```python
from build123d import *

# Parameters (mm, degrees)
SKIZZE2_R                            = 0.75
SCHNITT_LINEAR_AUSTRAGEN1_DEPTH      = 60.476886267
SKIZZE3_R                            = 3.5
SCHNITT_LINEAR_AUSTRAGEN2_DEPTH      = 25
SCHNITT_LINEAR_AUSTRAGEN3_DEPTH      = 60.476886267
SCHNITT_LINEAR_AUSTRAGEN3_DEPTH_BACK = 5
SKIZZE4_R                            = 6
SKIZZE5_W                            = 10
SKIZZE5_H                            = 60
SCHNITT_LINEAR_AUSTRAGEN4_DEPTH      = 60.476886435


with BuildPart() as part:
    # Skizze1 → Rotation1 (revolve)
    with BuildSketch(Plane.XY, mode=Mode.PRIVATE) as rotation1_sk:
        Polygon((0, 0), (-22.5, 0), (-27.5, 45), (0, 45), align=None)
    revolve(rotation1_sk.sketch.rotate(Axis((0, 0, 0), (0, 1, 0)), 270), axis=Axis((0, 0, 0), (0, 1, 0)))

    # Skizze2 → Schnitt-Linear austragen1 (cut, through all)
    with BuildSketch(Plane(origin=(0, 45, 0), x_dir=(1, 0, 0), z_dir=(0, 1, 0))):
        with Locations(Location((0, 0, 0), (0, 0, 270))):
            Circle(SKIZZE2_R)
    extrude(amount=-SCHNITT_LINEAR_AUSTRAGEN1_DEPTH, mode=Mode.SUBTRACT)

    # Skizze3 → Schnitt-Linear austragen2 (cut)
    with BuildSketch(Plane.XZ):
        with Locations(Location((0, 0, 0), (0, 0, 270))):
            Circle(SKIZZE3_R)
    extrude(amount=-SCHNITT_LINEAR_AUSTRAGEN2_DEPTH, mode=Mode.SUBTRACT)

    # Skizze4 → Schnitt-Linear austragen3 (cut, two sides: drawn at the far end of the back side and taken through both)
    with BuildSketch(Plane(origin=(0, 0, 0), x_dir=(0, 0, -1), z_dir=(1, 0, 0)).offset(-SCHNITT_LINEAR_AUSTRAGEN3_DEPTH_BACK)):
        with Locations(Location((0, 22.5, 0), (0, 0, 303.25844047))):
            Circle(SKIZZE4_R)
    extrude(amount=SCHNITT_LINEAR_AUSTRAGEN3_DEPTH + SCHNITT_LINEAR_AUSTRAGEN3_DEPTH_BACK, mode=Mode.SUBTRACT)

    # Skizze5 → Schnitt-Linear austragen4 (cut, through all)
    with BuildSketch(Plane(origin=(0, 45, 0), x_dir=(1, 0, 0), z_dir=(0, 1, 0))):
        with Locations((-26.5, 0)):
            Rectangle(SKIZZE5_W, SKIZZE5_H)
        with Locations((26.5, 0)):
            Rectangle(SKIZZE5_W, SKIZZE5_H)
    extrude(amount=-SCHNITT_LINEAR_AUSTRAGEN4_DEPTH, mode=Mode.SUBTRACT)


solid = part.part
```
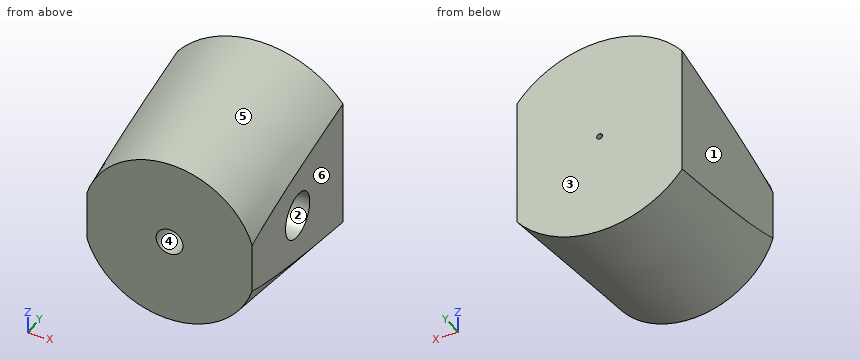
Input: part model. Units: mm. Frame: model coordinates. Face numbers are marked on the shaded views. A direction names the side the tool comes from. Coordinates: 2 decimals unless noted, no trailing zeros. Write each loop counter-clockwise with the first axis right and the second up, starting at its lowest first coordinate (ties: lowest second). Pieces come first, ordered by that corner, then holes. Notation, with made-up numbers: (60.5, 71) -> (105.5, 71) arc R19 cw to (105.5, 89) -> close; hole circle Ø10 at (15, 81). An arc over 180 degrees is marked (long way). Answer as a JSON object with one key per item and string values.
1. Section C-C on y = 42.5. Return the cut outline in (x, z).
Result set:
{"outline": "(-21.5, -16.7) arc R27.22 ccw to (21.5, -16.7) -> (21.5, 16.7) arc R27.22 ccw to (-21.5, 16.7) -> close; hole circle Ø1.5 at (0, 0)"}
2. First-contact query: P1, Ø4, axis at x = 16, y = 19, coming from the -Z side; P2, Ø9.5, axis at y = 22.5, z = 0, coming from the +X side; P3, Ø1, axis at x = -15.5, y = 34.5, coming from the -Z side. Flat tips, straight axial feed; report the tip coordinate or a pass-through.
Result set:
{"P1": "stops at z = -20.27", "P2": "stops at x = -5", "P3": "stops at z = -21.65"}
3. Section D-D on y = 22.5. Return the cut outline in (x, z).
Result set:
{"outline": "(-21.5, -12.76) arc R25 ccw to (21.5, -12.76) -> (21.5, -6) -> (-5, -6) -> (-5, 6) -> (21.5, 6) -> (21.5, 12.76) arc R25 ccw to (-21.5, 12.76) -> close"}
4. Mould query, pull axis X, two halves, no side actions, for the marked faces 3, 4, 5 and 6. Classes: released by +X, released by -X, zero draft, split by the parting line, or undercut.
Result set:
{"face 3": "zero draft", "face 4": "undercut", "face 5": "split by the parting line", "face 6": "released by +X"}
5. Material intervals for line 1 (X direction, y = 12, z = 0); line 2 (X direction, y = 33.25, z = 0); line 3 (Y direction, x = 8, z = 0), sorted ascending. Write a range as from..to.
Result set:
{"line 1": "x = -21.5..-3.5, 3.5..21.5", "line 2": "x = -21.5..-0.75, 0.75..21.5", "line 3": "y = 0..16.5, 28.5..45"}
6. Section A-A on z = 0. Return the cut outline in (x, y), then the cut area to 3 significant figures.
Result set:
{"outline": "(-21.5, 0) -> (-3.5, 0) -> (-3.5, 16.5) -> (-5, 16.5) -> (-5, 28.5) -> (-0.75, 28.5) -> (-0.75, 45) -> (-21.5, 45) -> close; (0.75, 28.5) -> (21.5, 28.5) -> (21.5, 45) -> (0.75, 45) -> close; (3.5, 0) -> (21.5, 0) -> (21.5, 16.5) -> (3.5, 16.5) -> close", "area": "1,480 mm2"}
7. Section B-B on x = 0. Return the cut outline in (y, z), then the cut area to 3 significant figures.
Result set:
{"outline": "(0, -22.5) -> (45, -27.5) -> (45, -0.75) -> (28.45, -0.75) arc R6 cw to (17.63, -3.5) -> (0, -3.5) -> close; (0, 3.5) -> (17.63, 3.5) arc R6 cw to (28.45, 0.75) -> (45, 0.75) -> (45, 27.5) -> (0, 22.5) -> close", "area": "1,990 mm2"}
8. Access query for the marked faces 1 and 2. Directions: +Z, -Z, +X, -X, +Y, -Y. A direction counts if a zero-diameter tool reaches every point of the face in a straight line with its end or side. Return the directions, or none.
Result set:
{"face 1": "+Z, -Z, -X, +Y, -Y", "face 2": "+X"}
